Part model, mm, in its own coordinate system. A direction names the side the tool comes from. Coordinates: 2 decimals unless noted, no trailing zeros. Loops run counter-clockwise (first coordinate to the right, second up) from the corner with the lowest first, then second, coordinate; pieces in that order, holes last. Notation, with made-up numbers: (-34.75, -23) - (-1.75, -23) arc R29 cw to (-1.75, 10) - close; hole circle Ø5 at (-11, 8.25). An arc over 180 degrees is marked (long way). Use a Markdown table: item, result. Add a question column.
1. Band-saw the part on B-B, the plane y = -19. Give the cut face in (x, z), plus the area to 3 significant figures.
2. Band-saw the part on C-C, the plane z = -14.25. Give the cut face in (x, y) (3 decimals), plus the area to 3 significant figures.
3. Band-saw the part on A-A, the plane y = -10.5. Give the cut face in (x, z), plus the area to 3 significant figures.
4. Pull direction Y, two halves, no side cores. Call faces 3 (the flat face through (53, -25.4, -1)), 4 (the cylindrical face through (2.905, -9.858, -1.252)), 5 (the flat face through (49.309, -14, -1)), 6 (the flat face through (28, 5.715, -13)): pulls with the +Y half, pulls with the -Y half, needs draft (parallel to the pull), parting line crosses it, or undercut.
5. Wall check: probe 1 along Z at (x, y) = (3, -1); probe 2 along X at (y, z) = (-13, -1.25); probe 3 along Y at (x, z) = (4, -12.25) (3 decimals). Give the ranges that are in metal, low to high. Write a range as [from, to].
6. Band-saw the part on D-D, the plane y = 1.5. Give the cut face in (x, z).
7. 3-axis set-ups, long thin cutter, end or side, ignore diameter. For faces 1 (the cylindrical face through (50.327, -17.279, -1.252)), 2 (the flat face through (3, -14, -2.54)): which of +Z, -Z, +X, -X, +Y, -Y reach the whole face in a straight line?
8. Drop flat-ended pins along their axis: pin 1 (4 mm diameter, centred on x = 52.852, z = -22.102, fed in from -Y); pin 2 (6 mm diameter, centred on x = 3.425, y = -17.385, fed in from -Z). Give the stop position or say it passes through.
from build123d import *

# Parameters (mm, degrees)
SKETCH1_W           = 56.15
SKETCH1_H           = 25.4
BOSS_EXTRUDE1_DEPTH = 2.54
SKETCH2_W           = 56.15
SKETCH2_H           = 25.4
BOSS_EXTRUDE2_DEPTH = 2.54
SKETCH3_R           = 2.400000018
CUT_EXTRUDE1_DEPTH  = 26.4
SKETCH11_W          = 56.15
SKETCH11_H          = 25.4
BOSS_EXTRUDE3_DEPTH = 5.715
SKETCH6_R           = 1.774
CUT_EXTRUDE3_DEPTH  = 9.255
CUT_EXTRUDE4_DEPTH  = 26.4


with BuildPart() as part:
    # Sketch1 → Boss-Extrude1 (new body)
    with BuildSketch(Plane(origin=(0, 0, 0), x_dir=(1, 0, 0), z_dir=(0, 1, 0))):
        with Locations((28.075, 12.7)):
            Rectangle(SKETCH1_W, SKETCH1_H)
    extrude(amount=-BOSS_EXTRUDE1_DEPTH)

    # Sketch2 → Boss-Extrude2 (add)
    with BuildSketch(Plane.XY):
        with Locations((28.075, -12.7)):
            Rectangle(SKETCH2_W, SKETCH2_H)
    extrude(amount=-BOSS_EXTRUDE2_DEPTH)

    # Sketch3 → Cut-Extrude1 (cut, through all)
    with BuildSketch(Plane.XY):
        with Locations((3.425, -7.515)):
            Circle(SKETCH3_R)
        with Locations((3.425, -17.385)):
            Circle(SKETCH3_R)
        with Locations((52.725, -7.515)):
            Circle(SKETCH3_R)
        with Locations((52.725, -17.385)):
            Circle(SKETCH3_R)
    extrude(amount=-CUT_EXTRUDE1_DEPTH, mode=Mode.SUBTRACT)

    # Sketch11 → Boss-Extrude3 (add)
    with BuildSketch(Plane(origin=(0, 0, 0), x_dir=(1, 0, 0), z_dir=(0, 1, 0))):
        with Locations((28.075, 12.7)):
            Rectangle(SKETCH11_W, SKETCH11_H)
    extrude(amount=BOSS_EXTRUDE3_DEPTH)

    # Sketch6 → Cut-Extrude3 (cut, through all)
    with BuildSketch(Plane.XZ.offset(2.54)):
        with Locations((52.852, -22.102)):
            Circle(SKETCH6_R)
        with Locations((52.852, -9.664)):
            Circle(SKETCH6_R)
        with Locations((3.298, -9.664)):
            Circle(SKETCH6_R)
        with Locations((3.298, -22.102)):
            Circle(SKETCH6_R)
    extrude(amount=-CUT_EXTRUDE3_DEPTH, mode=Mode.SUBTRACT)

    # Sketch7 → Cut-Extrude4 (cut, through all)
    with BuildSketch(Plane.XY):
        Polygon((49.308999982, -2.54), (6.841000018, -2.54), (6.841000018, -7.515), (6.841000018, -25.4), (49.308999982, -25.4), align=None)
    extrude(amount=-CUT_EXTRUDE4_DEPTH, mode=Mode.SUBTRACT)


solid = part.part
Geometry check:
| question | item | result |
|---|---|---|
| 1 | outline | (0, -2.54) - (1.65, -2.54) - (1.65, 0) - (0, 0) - close; (5.2, -2.54) - (6.84, -2.54) - (6.84, 0) - (5.2, 0) - close; (49.31, -2.54) - (50.95, -2.54) - (50.95, 0) - (49.31, 0) - close; (54.5, -2.54) - (56.15, -2.54) - (56.15, 0) - (54.5, 0) - close |
| 1 | area | 16.7 mm^2 |
| 2 | outline | (0, -2.54) - (56.15, -2.54) - (56.15, 5.715) - (0, 5.715) - close |
| 2 | area | 464 mm^2 |
| 3 | outline | (0, -2.54) - (6.84, -2.54) - (6.84, 0) - (0, 0) - close; (49.31, -2.54) - (56.15, -2.54) - (56.15, 0) - (49.31, 0) - close |
| 3 | area | 34.8 mm^2 |
| 4 | face 3 | pulls with the -Y half |
| 4 | face 4 | undercut |
| 4 | face 5 | needs draft |
| 4 | face 6 | pulls with the +Y half |
| 5 | probe 1 | z = [-25.4, -23.85], [-20.35, -11.41], [-7.92, 0] |
| 5 | probe 2 | x = [0, 6.84], [49.31, 56.15] |
| 5 | probe 3 | y = [-2.54, 5.715] |
| 6 | outline | (0, -25.4) - (56.15, -25.4) - (56.15, 0) - (0, 0) - close; hole circle Ø3.55 at (3.3, -22.1); hole circle Ø3.55 at (3.3, -9.66); hole circle Ø3.55 at (52.85, -22.1); hole circle Ø3.55 at (52.85, -9.66) |
| 7 | face 1 | +Z, -Z |
| 7 | face 2 | -Z, +X, -X, -Y |
| 8 | pin 1 | stops at y = -2.54 |
| 8 | pin 2 | stops at z = -2.54 |
